Part model, mm, in its own coordinate system. A direction names the side the tool comes from. Give positions to 0.01 mm unless a question says otherwise; leave off trailing zeros. Order: outer loops, then holes, each group sorted by start corner. A loop starts at its lowest first (then second) coordinate and runs counter-clockwise, first axis right, second up.
1. Slice it at B-B on z = 54. List the corners of the cut face in (x, y), and give its area (3 significant figures).
2. Slice it at D-D on z = 17. List the corners of the cut face in (x, y), and give its area (3 significant figures).
3. Probe line 1 (X direction, y = 5.75, z = 95); line 2 (Y direction, x = 111, z = 74); line 3 (Y direction, x = 123.5, z = 103). List the from-to ranges inside material, lowest first.
4. Slice it at A-A on y = 19.75. List the corners of the cut face in (x, z).
5. Which spindle directions (+Z, -Z, +X, -X, +Y, -Y) get a long thin tool onto all of the face, cutting with end or side? Do faces 5 (the flat face through (4, 7, 31)), 6 (the flat face through (6, 15, 63)), 7 (the flat face through (77, 4, 55)), 8 (the flat face through (149, 6, 55)). Say none if no direction does.
6. Drop flat-ended pins along their axis: pin 1 Ø3 at (x, z) = (115, 79.5) entering from +Y; pin 2 Ø6 at (y, z) = (7.5, 85) entering from +X; pin 3 Ø6 at (y, z) = (13.5, 84.5) entering from +X; pin 4 Ø4 at (x, y) = (67.5, 7.5) entering from +Z. Give the stop position or say it passes through.
7. Mould opens along X. For faces 1 (the flat face through (153, 2, 53)), 2 (the flat face through (4, 7, 77)), 3 (the flat face through (76, 6, 101)), 4 (the flat face through (5, 22, 47)) say: +X half, -X half, draft (parallel to the pull), parting line (faces both ways), or undercut.
8. Slice it at C-C on x = 59. List the corners of the cut face in (y, z), and give its area (3 significant figures).
Autodesk Inventor part; units mm, degrees
ref_plane "YZ Plane" through (0, 0, 0) normal (1, 0, 0) x (0, 1, 0)
ref_plane "XZ Plane" through (0, 0, 0) normal (0, 1, 0) x (-1, 0, 0)
ref_plane "XY Plane" through (0, 0, 0) normal (0, 0, 1) x (1, 0, 0)
sketch "Sketch1" plane through (0, 0, 0) normal (0, 1, 0) x (-1, 0, 0)
  line L0 (0, 0) -> (-153, 0)
  line L1 (-153, 0) -> (-153, 108)
  line L2 (-153, 108) -> (0, 108)
  line L3 (0, 108) -> (0, 0)
  dimension "d0" = 153
  dimension "d1" = 108
extrude "Extrusion1" add sketch "Sketch1" along normal blind 4
sketch "Sketch2" plane through (0, 4, 0) normal (0, 1, 0) x (1, 0, 0)
  line L0 (0, -108) -> (153, -108)
  line L1 (0, -108) -> (4, -108)
  line L2 (4, -108) -> (4, -104)
  line L3 (4, -104) -> (0, -104)
  line L4 (0, -104) -> (0, -108)
  line L5 (4, -104) -> (149, -104)
  line L6 (149, -104) -> (149, -4)
  line L7 (149, -4) -> (4, -4)
  line L8 (4, -4) -> (4, -104)
  line L9 (153, -108) -> (153, 0)
  line L10 (0, -108) -> (153, -108)
  line L11 (153, -108) -> (153, 0)
  line L12 (153, 0) -> (0, 0)
  line L13 (0, 0) -> (0, -108)
  line L14 (4, -104) -> (7, -104)
  line L15 (7, -104) -> (7, -101)
  line L16 (7, -101) -> (4, -101)
  line L17 (4, -101) -> (4, -104)
  line L18 (7, -101) -> (146, -101)
  line L19 (146, -101) -> (146, -7)
  line L20 (146, -7) -> (7, -7)
  line L21 (7, -7) -> (7, -101)
  dimension "d4" = 4
  dimension "d5" = 4
  dimension "d6" = 145
  dimension "d7" = 100
  dimension "d8" = 3
  dimension "d9" = 3
  dimension "d10" = 139
  dimension "d11" = 94
extrude "Extrusion2" add sketch "Sketch2" along normal blind 5 contours L8 L16 L15 L5 | L15 L16 L8 L7 L6 L5
sketch "Sketch3" plane through (0, 4, 0) normal (0, 1, 0) x (1, 0, 0)
  line L0 (0, 0) -> (0, -108)
  line L1 (0, -59) -> (4, -59)
  line L2 (4, -59) -> (4, -49)
  line L3 (4, -49) -> (0, -49)
  line L4 (0, -49) -> (0, -59)
  dimension "d14" = 4
  dimension "d15" = 10
extrude "Extrusion3" add sketch "Sketch3" along normal blind 18
sketch "Sketch4" plane through (4, 9, 49) normal (1, 0, 0) x (0, 0, -1)
  line L0 (0, 13) -> (-10, 13)
  circle A0 centre (-5, 13) radius 5
  point P0 (49, -9)
extrude "Extrusion4" cut sketch "Sketch4" against normal blind 18 contours A0 L0 picked at (-6.2475, 11.0971)
sketch "Sketch5" plane through (0, 9, 0) normal (0, 1, 0) x (1, 0, 0)
  line L0 (7, -101) -> (7, -7)
  line L1 (4, -45) -> (7, -45)
  line L2 (7, -45) -> (7, -63)
  line L3 (7, -63) -> (4, -63)
  line L4 (4, -63) -> (4, -45)
  point P0 (0, 0)
  dimension "d20" = 18
extrude "Extrusion5" add sketch "Sketch5" along normal blind 13
sketch "Sketch6" plane through (4, 22, 54) normal (-1, 0, 0) x (0, 0, 1)
  line L0 (-5, 0) -> (5, 0)
  circle A0 centre (0, 0) radius 5
  point P0 (-54, -22)
extrude "Extrusion6" cut sketch "Sketch6" against normal blind 13 contours L0 A0 picked at (0.9468, -1.3716)
properties part number "Golf Cart Mainboard Lid_3DPrint"
Data:
1. outline: (0, 0) - (153, 0) - (153, 4) - (149, 4) - (149, 9) - (146, 9) - (146, 4) - (7, 4) - (7, 17) - (0, 17) - close
1. area: 718 mm2
2. outline: (0, 0) - (153, 0) - (153, 4) - (149, 4) - (149, 9) - (146, 9) - (146, 4) - (7, 4) - (7, 9) - (4, 9) - (4, 4) - (0, 4) - close
2. area: 642 mm2
3. line 1: x = 4 to 7, 146 to 149
3. line 2: y = 0 to 4
3. line 3: y = 0 to 9
4. outline: (0, 49) - (4, 49) - (4, 45) - (7, 45) - (7, 49.53) - (0, 49.53) - close; (0, 58.47) - (7, 58.47) - (7, 63) - (4, 63) - (4, 59) - (0, 59) - close
5. face 5: -Z, -X, +Y
5. face 6: +Z, +X, -X, +Y
5. face 7: +Y
5. face 8: +Z, -Z, +X, +Y
6. pin 1: stops at y = 4
6. pin 2: stops at x = 149
6. pin 3: passes through
6. pin 4: stops at z = 104
7. face 1: +X half
7. face 2: -X half
7. face 3: undercut
7. face 4: draft
8. outline: (0, 0) - (4, 0) - (4, 4) - (9, 4) - (9, 7) - (4, 7) - (4, 101) - (9, 101) - (9, 104) - (4, 104) - (4, 108) - (0, 108) - close
8. area: 462 mm2
